Design review of the part built by this model. Coordinates are the model's own, in mm. Face numbers are marked on the shaded views. A direction names the side the tool comes from. Round coordinates to 2 decimals unless told otherwise and drop trailing zeros. Loops run counter-clockwise (first coordinate to the right, second up) from the corner with the lowest first, then second, coordinate; pieces in that order, holes last. Notation, with made-up numbers: M 2,78.5 L 32,78.5 A24 ccw 32,103.5 Z; hole C 59.25,68.5 d11. An arc over 180 degrees is marked long. Use a Markdown table: item, result.
Autodesk Inventor part; units mm, degrees
ref_plane "YZ Plane" through (0, 0, 0) normal (1, 0, 0) x (0, 1, 0)
ref_plane "XZ Plane" through (0, 0, 0) normal (0, 1, 0) x (-1, 0, 0)
ref_plane "XY Plane" through (0, 0, 0) normal (0, 0, 1) x (1, 0, 0)
sketch "Skizze1" plane through (0, 0, 0) normal (0, 0, 1) x (1, 0, 0)
  circle A0 centre (0, 0) radius 2.5
  circle A1 centre (0, 0) radius 4.5
  dimension "d0" = 5
  dimension "d1" = 9
extrude "Extrusion1" add sketch "Skizze1" along normal blind 30
sketch "Skizze2" plane through (0, 0, 30) normal (0, 0, 1) x (1, 0, 0)
  circle A0 centre (0, 0) radius 4.5
  circle A1 centre (0, 4.5) radius 2
  point P0 (1.95, 4.0556)
  point P1 (-1.95, 4.0556)
  dimension "d4" = 4
extrude "Extrusion2" add sketch "Skizze2" against normal blind 30 contours A0 A1 picked at (-0.7058, 5.0154)
sketch "Skizze3" plane through (0, 0, 30) normal (0, 0, 1) x (1, 0, 0)
  arc A0 (-1.95, 4.0556) -> (1.95, 4.0556) centre (0, 0) ccw
  arc A1 (1.95, 4.0556) -> (-1.95, 4.0556) centre (0, 4.5) ccw
  circle A2 centre (0, 0) radius 2.5
  circle A3 centre (0, 0) radius 8
  dimension "d7" = 16
extrude "Extrusion3" add sketch "Skizze3" along normal blind 1 contours A1 A0 | A3
properties part number "Motorcameralager"
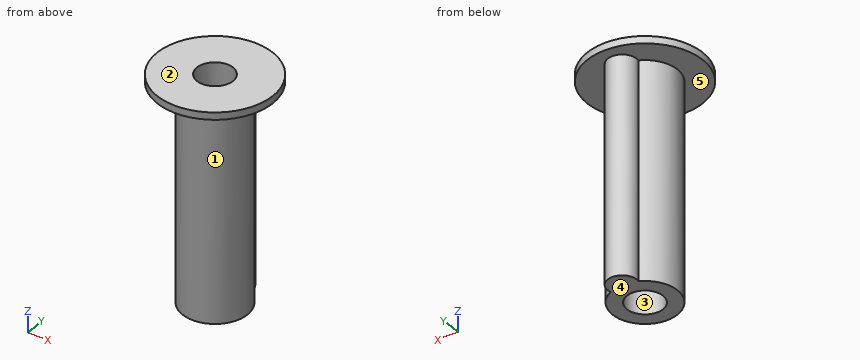
1. Wall thickness on line 1 along X through (y, z) = (-0.5, 19.5); line 2 along Z through (x, y) = (-6, -2); line 3 along X through (y, z) = (1.5, 28): over which ranges is each line inside the solid? List them lowest first. Write a range as from..to.
Check values:
| item | result |
|---|---|
| line 1 | x = -4.47..-2.45, 2.45..4.47 |
| line 2 | z = 30..31 |
| line 3 | x = -4.24..-2, 2..4.24 |
2. Take a section at B-B on x = 0. Give the boundary of the cut face in (y, z).
Check values:
| item | result |
|---|---|
| outline | M -8,30 L -4.5,30 L -4.5,0 L -2.5,0 L -2.5,31 L -8,31 Z; M 2.5,0 L 6.5,0 L 6.5,30 L 8,30 L 8,31 L 2.5,31 Z |
3. Machinability: for the marked faces 4 and 5, which of the approach directions +Z, -Z, +X, -X, +Y, -Y give a long, thin tool a straight path to every point of the face, cutting with its end or side? Answer none if there is none.
Check values:
| item | result |
|---|---|
| face 4 | -Z, +X, -X, +Y, -Y |
| face 5 | -Z |
4. Insertion check: pin 1 (2 mm diameter, centred on x = -1.5, z = 5.5, fed in from -Y); pin 2 (8 mm diameter, centred on x = 2, z = 23, fed in from +Y); pin 3 (6 mm diameter, centred on x = 4.5, z = 22, fed in from -Y); pin 4 (4.5 mm diameter, centred on x = 0, y = 0, fed in from +Z). Each pin has a flat end and moves straight along its axis. Give the tip position at first contact, or say it passes through.
Check values:
| item | result |
|---|---|
| pin 1 | stops at y = -4.47 |
| pin 2 | stops at y = 6.5 |
| pin 3 | stops at y = -4.24 |
| pin 4 | passes through |
5. Take a section at C-C on x = -3.25. Give the boundary of the cut face in (y, z), and give its area (3 significant figures).
Check values:
| item | result |
|---|---|
| outline | M -7.31,30 L -3.11,30 L -3.11,0 L 3.11,0 L 3.11,30 L 7.31,30 L 7.31,31 L -7.31,31 Z |
| area | 201 mm² |
6. Take a section at D-D on y = 4.5. Give the boundary of the cut face in (x, z).
Check values:
| item | result |
|---|---|
| outline | M -6.61,30 L -2,30 L -2,0 L 2,0 L 2,30 L 6.61,30 L 6.61,31 L -6.61,31 Z |
7. The part is to be moulded in two halves that separate along X. For the marked faces 1, 2 and 3, say which applies: pulls with the +X half, pulls with the -X half, needs draft (parallel to the pull), parting line crosses it, or undercut.
Check values:
| item | result |
|---|---|
| face 1 | parting line crosses it |
| face 2 | needs draft |
| face 3 | undercut |
8. Take a section at A-A on y = 0. Give the boundary of the cut face in (x, z).
Check values:
| item | result |
|---|---|
| outline | M -8,30 L -4.5,30 L -4.5,0 L -2.5,0 L -2.5,31 L -8,31 Z; M 2.5,0 L 4.5,0 L 4.5,30 L 8,30 L 8,31 L 2.5,31 Z |
